CAD build for the part. Positions are in the model's coordinates, mm. Face numbers are marked on the shaded views. Round coordinates to 2 decimals unless told otherwise and drop trailing zeros. Write each loop counter-clockwise with the first axis right and the second up, starting at its lowest first coordinate (ties: lowest second). Pieces come first, ordered by that corner, then holes. Notation, with made-up numbers: (26, 82.25) - (83, 82.25) arc R25 cw to (83, 119.25) - close; hole circle Ø9 at (15.25, -34). An arc over 180 degrees is marked (long way). Answer in a Markdown table with one row per item.
```python
from build123d import *

# Parameters (mm, degrees)
BOSS_EXTRUDE1_DEPTH                             = 2.032
SKETCH2_R                                       = 6.5405
CUT_EXTRUDE1_DEPTH                              = 21.32515872
CSK_FOR_M2_FLAT_HEAD_MACHINE_SCREW1_D           = 2
CSK_FOR_M2_FLAT_HEAD_MACHINE_SCREW1_CSINK_D     = 2.5
CSK_FOR_M2_FLAT_HEAD_MACHINE_SCREW1_CSINK_ANGLE = 90


with BuildPart() as part:
    # Sketch1 → Boss-Extrude1 (new body)
    with BuildSketch(Plane(origin=(0, 0, 0), x_dir=(1, 0, 0), z_dir=(0, 1, 0))):
        with BuildLine():
            ThreePointArc((4.932283688, 7.999686345), (-9.398, 0), (4.932283688, -7.999686345))
            ThreePointArc((4.932283688, -7.999686345), (17.907, 0), (4.932283688, 7.999686345))
        make_face()
    extrude(amount=BOSS_EXTRUDE1_DEPTH)

    # Sketch2 → Cut-Extrude1 (cut, through all)
    with BuildSketch(Plane(origin=(0, 2.032, 0), x_dir=(1, 0, 0), z_dir=(0, 1, 0))):
        with Locations(Location((0, 0, 0), (0, 0, 270))):
            Circle(SKETCH2_R)
    extrude(amount=-CUT_EXTRUDE1_DEPTH, mode=Mode.SUBTRACT)

    # CSK for M2 Flat Head Machine Screw1 (through all)
    with Locations(Plane(origin=(0, 2.032, 0), x_dir=(1, 0, 0), z_dir=(0, 1, 0))):
        with Locations((8.636, 6.985), (8.636, -6.985)):
            CounterSinkHole(CSK_FOR_M2_FLAT_HEAD_MACHINE_SCREW1_D / 2, CSK_FOR_M2_FLAT_HEAD_MACHINE_SCREW1_CSINK_D / 2, counter_sink_angle=CSK_FOR_M2_FLAT_HEAD_MACHINE_SCREW1_CSINK_ANGLE)


solid = part.part
```
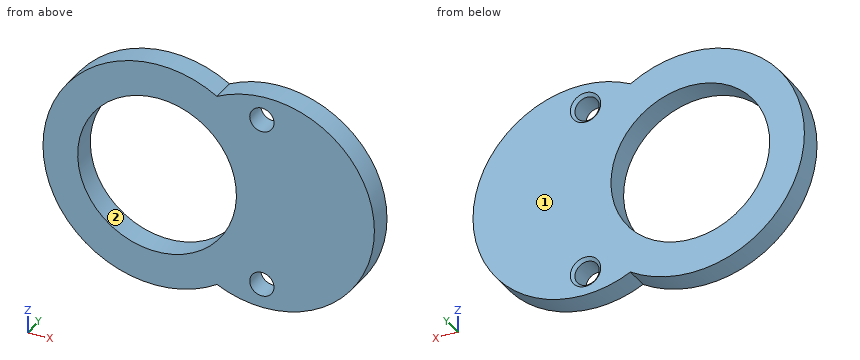
Q1. Flat gauge pins, fed straight in: pin 1 (1 mm diameter, centred on x = -3.5, y = 1, fed in from -Z); pin 2 (1.6 mm diameter, centred on x = 8.636, z = 6.985, fed in from +Y); pin 3 (5 mm diameter, centred on x = -1, z = -6, fed in from +Y). Where does each tip first touch, or does it go through?
Computed:
| item | result |
|---|---|
| pin 1 | stops at z = -8.91 |
| pin 2 | passes through |
| pin 3 | stops at y = 2.03 |
Q2. Saw through at A-A on z = 0. List the corners of the cut face in (x, y).
Computed:
| item | result |
|---|---|
| outline | (-9.4, 0) - (-6.54, 0) - (-6.54, 2.03) - (-9.4, 2.03) - close; (6.54, 0) - (17.91, 0) - (17.91, 2.03) - (6.54, 2.03) - close |
Q3. Saw through at C-C on y = 0.85. List the corners of the cut face in (x, z) (1 decimal), then the cut area to 3 significant figures.
Computed:
| item | result |
|---|---|
| outline | (4.9, -8) arc R9 ccw (long way) to (4.9, 8) arc R9.4 ccw (long way) to start; hole circle Ø13.1 at (0, 0); hole circle Ø2 at (8.6, -7); hole circle Ø2 at (8.6, 7) |
| area | 282 mm2 |
Q4. Drill centre lines: line 1 (X direction, y = 0.2, z = -7); line 2 (X direction, y = 0.45, z = 1.25); line 3 (Z direction, x = -3.75, y = 1.05). Where is each one in solid material? Low to high.
Computed:
| item | result |
|---|---|
| line 1 | x = -6.27 to 7.64, 9.64 to 14.54 |
| line 2 | x = -9.31 to -6.42, 6.42 to 17.82 |
| line 3 | z = -8.62 to -5.36, 5.36 to 8.62 |
Q5. Pull direction X, two halves, no side cores. Call the marked faces 1 and 2: released by +X, released by -X, zero draft, split by the parting line, or undercut.
Computed:
| item | result |
|---|---|
| face 1 | zero draft |
| face 2 | undercut |
Q6. Saw through at B-B on x = 0. List the corners of the cut face in (y, z).
Computed:
| item | result |
|---|---|
| outline | (0, -9.4) - (2.03, -9.4) - (2.03, -6.54) - (0, -6.54) - close; (0, 6.54) - (2.03, 6.54) - (2.03, 9.4) - (0, 9.4) - close |
Q7. Saw through at D-D on x = 8. Count the separate pieces of the cut face and the enclosed holes in it, then the cut area to 3 significant figures.
Computed:
| item | result |
|---|---|
| separate pieces | 3 |
| enclosed holes | 0 |
| area | 29.8 mm2 |
